Geometry: final body of the model. Coordinates: model frame, mm. A direction names the side the tool comes from. Give positions to 0.01 mm unless a question says otherwise; leave off trailing zeros. Write each loop counter-clockwise with the first axis right and the second up, starting at its lowest first coordinate (ties: lowest second). Pieces come first, ordered by that corner, then holes.
from build123d import *

# Parameters (mm, degrees)
SKETCH1_W           = 48.62
SKETCH1_H           = 22.26
BOSS_EXTRUDE1_DEPTH = 20
SKETCH2_R           = 1.876835713
BOSS_EXTRUDE2_DEPTH = 2.565394694
SKETCH3_R           = 11.694189136
BOSS_EXTRUDE3_DEPTH = 3


with BuildPart() as part:
    # Sketch1 → Boss-Extrude1 (new body)
    with BuildSketch(Plane.XY):
        Rectangle(SKETCH1_W, SKETCH1_H)
    extrude(amount=BOSS_EXTRUDE1_DEPTH)

    # Sketch2 → Boss-Extrude2 (add)
    with BuildSketch(Plane(origin=(0, 11.13, 0), x_dir=(1, 0, 0), z_dir=(0, 1, 0))):
        with Locations((-13.737467658, -9.398056281)):
            Circle(SKETCH2_R)
    extrude(amount=BOSS_EXTRUDE2_DEPTH)

    # Sketch3 → Boss-Extrude3 (add)
    with BuildSketch(Plane(origin=(0, 13.695394694, 0), x_dir=(1, 0, 0), z_dir=(0, 1, 0))):
        with Locations((-13.737467658, -9.398056281)):
            Circle(SKETCH3_R)
    extrude(amount=BOSS_EXTRUDE3_DEPTH)


solid = part.part
Q1. Section B-B on x = -17.5. Output: boundary loops of the cut face in (y, z), plus the area to 3 significant figures.
Filled sheet:
outline: (-11.13, 0) - (11.13, 0) - (11.13, 20) - (-11.13, 20) - close; (13.7, -1.67) - (16.7, -1.67) - (16.7, 20.47) - (13.7, 20.47) - close
area: 512 mm2
Q2. Section C-C on y = 10.25. Output: boundary loops of the cut face in (x, z).
Filled sheet:
outline: (-24.31, 0) - (24.31, 0) - (24.31, 20) - (-24.31, 20) - close
Q3. Pull-direction query (Y, two-part tool) for faces 1 (the flat face through (0, 0, 20)), 2 (the flat face through (-14, 13.695, 12)), 3 (the flat face through (-14, 16.695, 9)); classes: released by +Y, released by -Y, zero draft, split by the parting line, or undercut.
Filled sheet:
face 1: zero draft
face 2: undercut
face 3: released by +Y
Q4. Access query for faces 4 (the cylindrical face through (-2.935, 15.174, 13.877)), 5 (the flat face through (-24.31, 0, 10)), 6 (the flat face through (0, 0, 0)), 7 (the cylindrical face through (-13.982, 12.395, 7.537)). Directions: +Z, -Z, +X, -X, +Y, -Y. A direction counts if a zero-diameter tool reaches every point of the face in a straight line with its end or side. Return the directions, or none.
Filled sheet:
face 4: +Y
face 5: +Z, -Z, -X, -Y
face 6: -Z, +X, -X, -Y
face 7: none
Q5. Section D-D on x = 4. Output: boundary loops of the cut face in (y, z), plus the area to 3 significant figures.
Filled sheet:
outline: (-11.13, 0) - (11.13, 0) - (11.13, 20) - (-11.13, 20) - close
area: 445 mm2
Q6. Pin query (flat end, axial travel): P1, Ø6.5, axis at x = -7, y = 5, coming from the +Z side; P2, Ø10, axis at y = -1, z = 14.5, coming from the -X side; P3, Ø10, axis at x = -16, y = -4, coming from the -Z side. Return the tip coordinate at first contact, or that it passes through.
Filled sheet:
P1: stops at z = 20
P2: stops at x = -24.31
P3: stops at z = 0
Q7. Ray query, line 1 along Y through (x, z) = (-6, 10.5); line 2 along X through (y, z) = (-3.5, 13.75); line 3 along Y through (x, z) = (16.5, 7.25). Return the intervals inside material, ascending.
Filled sheet:
line 1: y = -11.13 to 11.13, 13.7 to 16.7
line 2: x = -24.31 to 24.31
line 3: y = -11.13 to 11.13
Q8. Section A-A on z = 12. Output: boundary loops of the cut face in (x, y).
Filled sheet:
outline: (-25.14, 13.7) - (-2.34, 13.7) - (-2.34, 16.7) - (-25.14, 16.7) - close; (-24.31, -11.13) - (24.31, -11.13) - (24.31, 11.13) - (-24.31, 11.13) - close
